from build123d import *

# Parameters (mm, degrees)
F0_W     = 250
F0_H     = 112
F1_DEPTH = 35
F2_R     = 8
F3_DEPTH = 400
F4_R     = 12.5
F5_DEPTH = 25
F6_R     = 2
F7_DEPTH = 6.1


with BuildPart() as f1:
    # F0 (on Front) → F1 (new body)
    with BuildSketch(Plane.XZ):
        with Locations((0, 7.5)):
            Rectangle(F0_W, F0_H)
        with BuildLine():
            Line((50, -18.5), (-50, -18.5))
            ThreePointArc((-50, -18.5), (-68.5, 0), (-50, 18.5))
            Line((-50, 18.5), (50, 18.5))
            ThreePointArc((50, 18.5), (68.5, 0), (50, -18.5))
        make_face(mode=Mode.SUBTRACT)
    extrude(amount=F1_DEPTH)

    # F2 (on face) → F3 (cut)
    with BuildSketch(Plane.XY.offset(63.5)):
        with Locations((-100, -17.5)):
            Circle(F2_R)
        with Locations((100, -17.5)):
            Circle(F2_R)
    extrude(amount=-F3_DEPTH, mode=Mode.SUBTRACT)

    # F4 (on face) → F5 (cut)
    with BuildSketch(Plane.XY.offset(63.5)):
        with Locations((0, -17.5)):
            Circle(F4_R)
    extrude(amount=-F5_DEPTH, mode=Mode.SUBTRACT)

    # F6 (on face) → F7 (cut)
    with BuildSketch(Plane.XY.offset(-18.5)):
        with Locations((-42.5, -4.5)):
            Circle(F6_R)
        with Locations((-42.5, -30.5)):
            Circle(F6_R)
        with Locations((42.5, -4.5)):
            Circle(F6_R)
        with Locations((42.5, -30.5)):
            Circle(F6_R)
    extrude(amount=-F7_DEPTH, mode=Mode.SUBTRACT)


solid = f1.part
Source: CAD feature listing. Evaluate the final solid. Frame: model axes, mm. A direction names the side the tool comes from. Round coordinates to 2 decimals unless told otherwise and drop trailing zeros. Loops run counter-clockwise (first coordinate to the right, second up) from the corner with the lowest first, then second, coordinate; pieces in that order, holes last. Notation, with made-up numbers: M 70,-32.75 L 76,-32.75 A16 cw 76,-23.75 Z; hole C 21.25,58 d7. An arc over 180 degrees is marked long. Return JSON: item names as keys, results as strings. Group by question number.
1. Reachability of faces 1 (the face through (-2.71, -29.703, 51.175)), 2 (the face through (-68.496, -17.255, -0.407)), 3 (the face through (-2, 0, 21)) from +Z, -Z, +X, -X, +Y, -Y: full face, straight path, thin tool, end or side. Return the list, or none.
2. Section query D-D on z = 41. Output: boundary loops of the cut face in (x, y), and give its area (3 significant figures).
3. Section query C-C on z = 14.5. Output: boundary loops of the cut face in (x, y), and give its area (3 significant figures).
4. Section query A-A on x = 0. Output: boundary loops of the cut face in (y, z), and give its area (3 significant figures).
5. Mould query, pull axis X, two halves, no side actions, for faces 4 (the face through (68.496, -17.255, 0.407)), 5 (the face through (125, -17, 7)), 6 (the face through (-2, -35, 21)), 7 (the face through (-125, -17, 7)). Classes: released by +X, released by -X, zero draft, split by the parting line, or undercut.
6. Material intervals for line 1 along Y through (x, z) = (42.5, -22); line 2 along Z through (x, y) = (16.5, -6); line 3 along Z through (x, y) = (-10.5, -21), sorted ascending. Write a range as from..to.
7. Section query B-B on y = -15. Output: boundary loops of the cut face in (x, z), and give its area (3 significant figures).
Checks:
{
 "1": {"face 1": "+Z", "face 2": "+Y, -Y", "face 3": "+Z, -Z, +X, -X, +Y"},
 "2": {"outline": "M -125,-35 L 125,-35 L 125,0 L -125,0 Z; hole C -100,-17.5 d16; hole C 0,-17.5 d25; hole C 100,-17.5 d16", "area": "7,860 mm²"},
 "3": {"outline": "M -125,-35 L -61.49,-35 L -61.49,0 L -125,0 Z; M 61.49,-35 L 125,-35 L 125,0 L 61.49,0 Z; hole C -100,-17.5 d16; hole C 100,-17.5 d16", "area": "4,040 mm²"},
 "4": {"outline": "M -35,-48.5 L 0,-48.5 L 0,-18.5 L -35,-18.5 Z; M -35,18.5 L 0,18.5 L 0,63.5 L -5,63.5 L -5,38.5 L -30,38.5 L -30,63.5 L -35,63.5 Z", "area": "2,000 mm²"},
 "5": {"face 4": "undercut", "face 5": "released by +X", "face 6": "zero draft", "face 7": "released by -X"},
 "6": {"line 1": "y = -35..-32.5, -28.5..-6.5, -2.5..0", "line 2": "z = -48.5..-18.5, 18.5..63.5", "line 3": "z = -48.5..-18.5, 18.5..38.5"},
 "7": {"outline": "M -125,-48.5 L -107.6,-48.5 L -107.6,63.5 L -125,63.5 Z; M -92.4,-48.5 L 92.4,-48.5 L 92.4,63.5 L 12.25,63.5 L 12.25,38.5 L -12.25,38.5 L -12.25,63.5 L -92.4,63.5 Z; M 107.6,-48.5 L 125,-48.5 L 125,63.5 L 107.6,63.5 Z; hole M -50,-18.5 L 50,-18.5 A18.5 ccw 50,18.5 L -50,18.5 A18.5 ccw Z", "area": "19,200 mm²"}
}
